Part model, mm, in its own coordinate system. A direction names the side the tool comes from. Coordinates: 2 decimals unless noted, no trailing zeros. Order: outer loops, then holes, each group sorted by start corner. A loop starts at its lowest first (then second) coordinate and runs counter-clockwise, first axis right, second up. Notation, with made-up numbers: (48.5, -3) - (88.5, -3) arc R12 cw to (88.5, 6) - close; hole circle Ø1 at (26, 6). An arc over 180 degrees is marked (long way). Use a Markdown table: item, result. Add a question column.
1) Tool access for faces 5 (the face through (8.874, 16.438, -1.165)), 6 (the face through (-5.3, 13.1, -6.9)), 7 (the face through (8, 0.7, 5)): list every direction of +Z, -Z, +X, -X, +Y, -Y with a clear straight run to the whole face (end or side of a thin tool).
2) Wall check: L1, parallel to X at y = 0.5, z = 1.25; L2, parallel to X at y = 8.75, z = 0.25; L3, parallel to Y at x = 4.5, z = -8.75. Give the ranges that are in metal, low to high. Write a range as [from, to].
3) Saw through at B-B on z = 1.25. Count the separate pieces of the cut face and the enclosed holes in it, then the cut area to 3 significant figures.
4) Two-plate mould, pull along Z, no slides. Class faces 1 (the face through (0.16, 1.14, -12.24)), 2 (the face through (8.874, 6.037, -1.165)), 3 (the face through (-12.768, 0.345, 2.438)), 4 (the face through (-10, 1.6, 0)): +Z half, -Z half, draft (parallel to the pull), parting line (faces both ways), or undercut.
5) Saw through at C-C on y = 11.75. List the corners of the cut face in (x, z), then the cut area to 3 significant figures.
6) Saw through at A-A on y = 4.5. List the corners of the cut face in (x, z).
7) Drop flat-ended pins along their axis: P1, Ø3, axis at x = -10.82, z = 2, coming from the -Y side; P2, Ø1.5, axis at x = 0, z = -11, coming from the +Y side; P3, Ø4, axis at y = 4.5, z = 2.5, coming from the -X side; P4, Ø3, axis at x = 5.5, z = 6, coming from the +Y side. Give the stop position or say it passes through.
```python
from build123d import *

# Parameters (mm, degrees)
SKETCH_1_R          = 15
EXTRUDE_1_DEPTH     = 1.6
SKETCH_2_R          = 8.95
EXTRUDE_2_DEPTH     = 16
SKETCH_3_R          = 8
CUT_EXTRUDE_1_DEPTH = 28.563744303
FILLET_1_R          = 2
MM_1_D              = 2.5
SKETCH_6_R          = 2
CUT_EXTRUDE_2_DEPTH = 0.7
CUT_EXTRUDE_START   = -7
SKETCH_7_R          = 8.95
SKETCH_7_R_2        = 8.7
CUT_EXTRUDE_3_DEPTH = 5
CHAMFER_1_SIZE      = 0.3


with BuildPart() as part:
    # 草图1 → 凸台-拉伸1 (new body)
    with BuildSketch(Plane(origin=(0, 0, 0), x_dir=(1, 0, 0), z_dir=(0, 1, 0))):
        with Locations(Location((0, 0, 0), (0, 0, 270))):
            Circle(SKETCH_1_R)
    extrude(amount=EXTRUDE_1_DEPTH)

    # 草图2 → 凸台-拉伸2 (add)
    with BuildSketch(Plane(origin=(0, 1.6, 0), x_dir=(1, 0, 0), z_dir=(0, 1, 0))):
        with Locations(Location((0, 0, 0), (0, 0, 270))):
            Circle(SKETCH_2_R)
    extrude(amount=EXTRUDE_2_DEPTH)

    # 草图3 → 切除-拉伸1 (cut, through all)
    with BuildSketch(Plane(origin=(0, 0, 0), x_dir=(-1, 0, 0), z_dir=(0, -1, 0))):
        with Locations(Location((0, 0, 0), (0, 0, 90))):
            Circle(SKETCH_3_R)
    extrude(amount=-CUT_EXTRUDE_1_DEPTH, mode=Mode.SUBTRACT)

    # 圆角1
    fillet_1_edges = [part.edges().sort_by_distance(p)[0] for p in [
        (0, 0, 8),
    ]]
    fillet(fillet_1_edges, radius=FILLET_1_R)

    # 大小mm 暗销孔1 (through all)
    with Locations(Plane(origin=(0, 1.6, 0), x_dir=(1, 0, 0), z_dir=(0, 1, 0))):
        with Locations((0, 11), (9.573912655, -5.416659161), (-10.815803983, -2.00459078)):
            Hole(MM_1_D / 2)

    # 草图6 → 切除-拉伸2 (cut)
    with BuildSketch(Plane(origin=(0, 0, 0), x_dir=(-1, 0, 0), z_dir=(0, -1, 0))):
        with Locations(Location((0, 11, 0), (0, 0, 90))):
            Circle(SKETCH_6_R)
        with Locations(Location((10.815803983, -2.00459078, 0), (0, 0, 90))):
            Circle(SKETCH_6_R)
        with Locations(Location((-9.573912655, -5.416659161, 0), (0, 0, 90))):
            Circle(SKETCH_6_R)
    extrude(amount=-CUT_EXTRUDE_2_DEPTH, mode=Mode.SUBTRACT)

    # 草图7 → 切除-拉伸3 (cut)
    with BuildSketch(Plane(origin=(0, 17.6, 0), x_dir=(1, 0, 0), z_dir=(0, 1, 0)).offset(CUT_EXTRUDE_START)):
        with Locations(Location((0, 0, 0), (0, 0, 270))):
            Circle(SKETCH_7_R)
        with Locations(Location((0, 0, 0), (0, 0, 270))):
            Circle(SKETCH_7_R_2, mode=Mode.SUBTRACT)
    extrude(amount=CUT_EXTRUDE_3_DEPTH, mode=Mode.SUBTRACT)

    # 倒角1
    chamfer_1_edges = [part.edges().sort_by_distance(p)[0] for p in [
        (0, 17.6, 8),
        (0, 0, -15),
        (0, 1.6, -15),
        (0, 17.6, -8.95),
    ]]
    chamfer(chamfer_1_edges, length=CHAMFER_1_SIZE)


solid = part.part
```
Results are:
| question | item | result |
|---|---|---|
| 1 | face 5 | +Y |
| 1 | face 6 | none |
| 1 | face 7 | -Y |
| 2 | L1 | [-14.95, -12.67], [-8.96, -8.59], [8.59, 14.95] |
| 2 | L2 | [-8.95, -8], [8, 8.95] |
| 2 | L3 | [0.01, 1.6] |
| 3 | separate pieces | 3 |
| 3 | enclosed holes | 0 |
| 3 | area | 44.3 mm2 |
| 4 | face 1 | undercut |
| 4 | face 2 | parting line |
| 4 | face 3 | undercut |
| 4 | face 4 | draft |
| 5 | outline | circle Ø17.4 at (0, 0); hole circle Ø16 at (0, 0) |
| 5 | area | 36.7 mm2 |
| 6 | outline | circle Ø17.9 at (0, 0); hole circle Ø16 at (0, 0) |
| 7 | P1 | y = 0.7 |
| 7 | P2 | through |
| 7 | P3 | x = -8.94 |
| 7 | P4 | y = 17.6 |
